Source: three-view drawing plus pictorial views. Frame: mm from the lowest corner of the part. Coordinates: 2 decimals unless noted, no trailing zeros. Loops run counter-clockwise (first coordinate to the right, second up) from the corner with the lowest first, then second, coordinate; pieces in that order, holes last. Notation, with made-up numbers: (43, 48) - (86, 48) arc R33 ccw to (86, 76) - close; hole circle Ø5 at (35, 62.25). An arc over 180 degrees is marked (long way). Return JSON: item names as keys, results as strings.
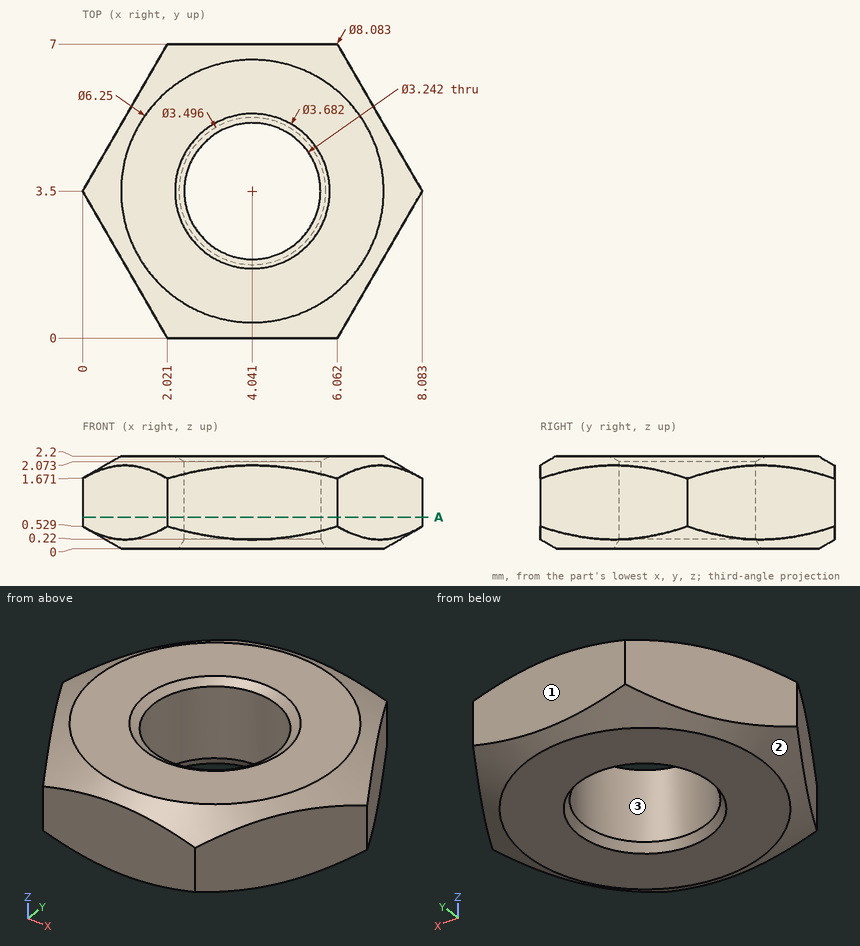
Item 1: Section query A-A, the plane z = 0.75. Return loops of the section in (x, y).
Worked out:
{"outline": "(0, 3.5) - (2.02, 0) - (6.06, 0) - (8.08, 3.5) - (6.06, 7) - (2.02, 7) - close; hole circle Ø3.24 at (4.04, 3.5)"}
Item 2: Mould query, pull axis X, two halves, no side actions, for the marked faces 1, 2 and 3. Classes: +X half, -X half, draft (parallel to the pull), parting line (faces both ways), or undercut.
Worked out:
{"face 1": "draft", "face 2": "parting line", "face 3": "undercut"}
Item 3: Ray query, probe 1 along Y at (x, z) = (4.25, 1.65); probe 2 along X at (y, z) = (4.5, 1.3) (1 decimal); probe 3 along X at (y, z) = (4.5, 2) (1 decimal). Return the intervals inside material, ascending. Write a range as from..to.
Worked out:
{"probe 1": "0..1.89, 5.11..7", "probe 2": "0.6..2.8, 5.3..7.5", "probe 3": "0.7..2.8, 5.3..7.4"}
